Part model, mm, in its own coordinate system. A direction names the side the tool comes from. Round coordinates to 2 decimals unless told otherwise and drop trailing zeros. Order: outer loops, then holes, each group sorted by start corner. A loop starts at its lowest first (then second) coordinate and runs counter-clockwise, first axis right, second up. Notation, with made-up numbers: (19.5, 45.5) -> (51.5, 45.5) arc R13 cw to (51.5, 64.5) -> close; hole circle Ø1 at (44.25, -26.75). An arc over 180 degrees is marked (long way). Answer as a JSON object with one key per item and string values. Group by question number.
```python
from build123d import *

# Parameters (mm, degrees)
SKETCH1_W           = 15
SKETCH1_H           = 77.5
BOSS_EXTRUDE1_DEPTH = 10
SKETCH3_R           = 1
CUT_EXTRUDE1_DEPTH  = 10
SKETCH4_R           = 1
CUT_EXTRUDE2_DEPTH  = 10
SKETCH5_R           = 1.5
CUT_EXTRUDE3_DEPTH  = 5


with BuildPart() as part:
    # Sketch1 → Boss-Extrude1 (new body)
    with BuildSketch(Plane(origin=(0, 0, 0), x_dir=(0, 0, -1), z_dir=(1, 0, 0))):
        with Locations((7.5, 38.75)):
            Rectangle(SKETCH1_W, SKETCH1_H)
    extrude(amount=BOSS_EXTRUDE1_DEPTH)

    # Sketch3 → Cut-Extrude1 (cut)
    with BuildSketch(Plane(origin=(0, 77.5, 0), x_dir=(1, 0, 0), z_dir=(0, 1, 0))):
        with Locations((2, 13)):
            Circle(SKETCH3_R)
        with Locations((8, 13)):
            Circle(SKETCH3_R)
        with Locations((8, 2)):
            Circle(SKETCH3_R)
        with Locations((2, 2)):
            Circle(SKETCH3_R)
    extrude(amount=-CUT_EXTRUDE1_DEPTH, mode=Mode.SUBTRACT)

    # Sketch4 → Cut-Extrude2 (cut)
    with BuildSketch(Plane(origin=(0, 0, 0), x_dir=(-1, 0, 0), z_dir=(0, -1, 0))):
        with Locations((-8, 2)):
            Circle(SKETCH4_R)
        with Locations((-8, 13)):
            Circle(SKETCH4_R)
        with Locations((-2, 13)):
            Circle(SKETCH4_R)
        with Locations((-2, 2)):
            Circle(SKETCH4_R)
    extrude(amount=-CUT_EXTRUDE2_DEPTH, mode=Mode.SUBTRACT)

    # Sketch5 → Cut-Extrude3 (cut)
    with BuildSketch(Plane(origin=(10, 0, 0), x_dir=(0, 0, -1), z_dir=(1, 0, 0))):
        with Locations((6, 61.5)):
            Circle(SKETCH5_R)
        with Locations((6, 54.5)):
            Circle(SKETCH5_R)
    extrude(amount=-CUT_EXTRUDE3_DEPTH, mode=Mode.SUBTRACT)


solid = part.part
```
Q1. Band-saw the part on D-D (x = 2). List the corners of the cut face in (y, z), plus the area to 3 significant figures.
Q2. Two-plate mould, pull along X, no slides. Class faces 1 (the flat face through (0, 39, -7)), 2 (the flat face through (8, 67.5, -2)), 3 (the cylindrical face through (8, 73, -12)), 4 (the flat face through (5, 0, -7)): +X half, -X half, draft (parallel to the pull), parting line (faces both ways), or undercut.
Q3. Wall check: line 1 (X direction, y = 70.5, z = -2); line 2 (Z direction, x = 8, y = 7.5); line 3 (Y direction, x = 8.95, z = -6). Give the ranges that are in metal, low to high. Write a range as [from, to].
Q4. Band-saw the part on A-A (x = 8). List the corners of the cut face in (y, z), plus the area to 3 significant figures.
Q5. Band-saw the part on C-C (y = 61.5). List the corners of the cut face in (x, z).
Q6. Drop flat-ended pins along their axis: pin 1 Ø1.2 at (x, z) = (2, -2) entering from -Y; pin 2 Ø2.5 at (y, z) = (61.5, -6) entering from +X; pin 3 Ø0.6 at (x, z) = (2, -13) entering from +Y. Give the stop position or say it passes through.
Q7. Which spindle directions (+Z, -Z, +X, -X, +Y, -Y) get a long thin tool onto all of the face, cutting with end or side? Do faces 5 (the cylindrical face through (7.2, 72.6, -1.4)), 6 (the cylindrical face through (8, 5, -12)), 7 (the flat face through (5, 62, -6)). Say none if no direction does.
Q8. Band-saw the part on B-B (z = -13). List the corners of the cut face in (x, y), plus the area to 3 significant figures.
Completed:
{
 "1": {"outline": "(0, -15) -> (77.5, -15) -> (77.5, -14) -> (67.5, -14) -> (67.5, -12) -> (77.5, -12) -> (77.5, -3) -> (67.5, -3) -> (67.5, -1) -> (77.5, -1) -> (77.5, 0) -> (0, 0) -> (0, -1) -> (10, -1) -> (10, -3) -> (0, -3) -> (0, -12) -> (10, -12) -> (10, -14) -> (0, -14) -> close", "area": "1,080 mm2"},
 "2": {"face 1": "-X half", "face 2": "undercut", "face 3": "undercut", "face 4": "draft"},
 "3": {"line 1": "[0, 1], [3, 7], [9, 10]", "line 2": "[-15, -14], [-12, -3], [-1, 0]", "line 3": "[0, 53], [56, 60], [63, 77.5]"},
 "4": {"outline": "(0, -15) -> (77.5, -15) -> (77.5, -14) -> (67.5, -14) -> (67.5, -12) -> (77.5, -12) -> (77.5, -3) -> (67.5, -3) -> (67.5, -1) -> (77.5, -1) -> (77.5, 0) -> (0, 0) -> (0, -1) -> (10, -1) -> (10, -3) -> (0, -3) -> (0, -12) -> (10, -12) -> (10, -14) -> (0, -14) -> close; hole circle Ø3 at (54.5, -6); hole circle Ø3 at (61.5, -6)", "area": "1,070 mm2"},
 "5": {"outline": "(0, -15) -> (10, -15) -> (10, -7.5) -> (5, -7.5) -> (5, -4.5) -> (10, -4.5) -> (10, 0) -> (0, 0) -> close"},
 "6": {"pin 1": "y = 10", "pin 2": "x = 5", "pin 3": "y = 67.5"},
 "7": {"face 5": "+Y", "face 6": "-Y", "face 7": "+X"},
 "8": {"outline": "(0, 0) -> (1, 0) -> (1, 10) -> (3, 10) -> (3, 0) -> (7, 0) -> (7, 10) -> (9, 10) -> (9, 0) -> (10, 0) -> (10, 77.5) -> (9, 77.5) -> (9, 67.5) -> (7, 67.5) -> (7, 77.5) -> (3, 77.5) -> (3, 67.5) -> (1, 67.5) -> (1, 77.5) -> (0, 77.5) -> close", "area": "695 mm2"}
}
